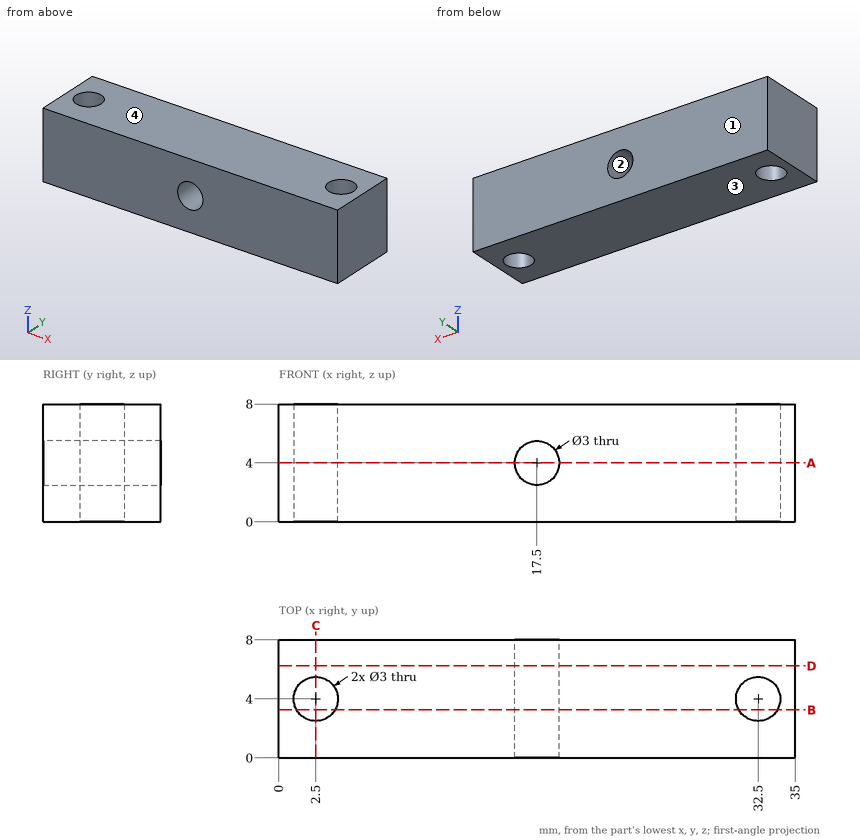
The figure shows three views and two pictorial views of one solid part (mm, origin at its lowest corner). Answer the questions. Round coordinates to 2 decimals unless told otherwise and drop trailing zeros. Loops run counter-clockwise (first coordinate to the right, second up) from the corner with the lowest first, then second, coordinate; pieces in that order, holes last. Notation, with made-up numbers: M -2.75,20 L 15.25,20 A11 ccw 15.25,30 Z; hole C 30,-1.5 d7. An arc over 180 degrees is marked long. Return JSON: item names as keys, results as strings.
Q1. Find section B-B, the plane y = 3.25. Determine the outline of the cut face in (x, z).
Results list:
{"outline": "M 0,0 L 1.2,0 L 1.2,8 L 0,8 Z; M 3.8,0 L 31.2,0 L 31.2,8 L 3.8,8 Z; M 33.8,0 L 35,0 L 35,8 L 33.8,8 Z; hole C 17.5,4 d3"}
Q2. Find the intervals of material crossed by line 1 along X through (y, z) = (2.25, 4); line 2 along Y through (x, z) = (2.5, 2); line 3 along X through (y, z) = (5.25, 4.25), in increasing order. Write a range as from..to.
Results list:
{"line 1": "x = 0..16, 19..35", "line 2": "y = 0..2.5, 5.5..8", "line 3": "x = 0..1.67, 3.33..16.02, 18.98..31.67, 33.33..35"}
Q3. Find section C-C, the plane x = 2.5. Determine the outline of the cut face in (y, z), plus the area to 3 significant figures.
Results list:
{"outline": "M 0,0 L 2.5,0 L 2.5,8 L 0,8 Z; M 5.5,0 L 8,0 L 8,8 L 5.5,8 Z", "area": "40.0 mm2"}
Q4. Find section D-D, the plane y = 6.25. Determine the outline of the cut face in (x, z), plus the area to 3 significant figures.
Results list:
{"outline": "M 0,0 L 35,0 L 35,8 L 0,8 Z; hole C 17.5,4 d3", "area": "273 mm2"}
Q5. Find section A-A, the plane z = 4. Determine the outline of the cut face in (x, y).
Results list:
{"outline": "M 0,0 L 16,0 L 16,8 L 0,8 Z; M 19,0 L 35,0 L 35,8 L 19,8 Z; hole C 2.5,4 d3; hole C 32.5,4 d3"}
Q6. The mould has two halves that part along Z. Classify the marked faces 1, 2, 3 and 4: released by +Z, released by -Z, zero draft, split by the parting line, or undercut.
Results list:
{"face 1": "zero draft", "face 2": "undercut", "face 3": "released by -Z", "face 4": "released by +Z"}
Q7. This flat-tipped pin is pushed along its axis until it touches: pin 1 Ø2 at (y, z) = (2, 4.5) entering from -X. Where does it stop, or does it pass through?
Results list:
{"pin 1": "stops at x = 0"}
